Geometry: final body of the model. Coordinates: model frame, mm. A direction names the side the tool comes from. Coordinates: 2 decimals unless noted, no trailing zeros. Write each loop counter-clockwise with the first axis right and the second up, starting at its lowest first coordinate (ties: lowest second). Pieces come first, ordered by that corner, then holes.
Autodesk Inventor part; units mm, degrees
ref_plane "YZ Plane" through (0, 0, 0) normal (1, 0, 0) x (0, 1, 0)
ref_plane "XZ Plane" through (0, 0, 0) normal (0, 1, 0) x (-1, 0, 0)
ref_plane "XY Plane" through (0, 0, 0) normal (0, 0, 1) x (1, 0, 0)
sketch "Sketch1" plane through (0, 0, 0) normal (0, 0, 1) x (1, 0, 0)
  circle A0 centre (0, 0) radius 5
  line L0 (0, 0) -> (25, 0) construction
  line L1 (0, -10) -> (25, -10)
  line L2 (25, 10) -> (0, 10)
  arc A1 (0, 10) -> (0, -10) centre (0, 0) ccw
  arc A2 (25, -10) -> (25, 10) centre (25, 0) ccw construction
  line L3 (25, 10) -> (25, -10)
  point P0 (12.5, 0)
  dimension "d0" = 10
  dimension "d1" = 5
  dimension "d2" = 25
extrude "Extrusion1" add sketch "Sketch1" along normal blind 4
sketch "Sketch2" plane through (0, -10, 0) normal (0, -1, 0) x (1, 0, 0)
  line L0 (0, 4) -> (25, 4)
  line L1 (25, 4) -> (10, 4)
  line L2 (10, 4) -> (10, 19)
  line L3 (10, 19) -> (25, 19)
  line L4 (25, 19) -> (25, 4)
  line L5 (17.5, 19) -> (17.5, 4) construction
  circle A0 centre (17.5, 11.5) radius 4
  point P0 (0, 0)
  dimension "d5" = 8
  dimension "d6" = 15
  dimension "d7" = 15
extrude "Extrusion2" add sketch "Sketch2" against normal up to surface (20 mm away)
fillet "Fillet1" radius 7 2 edges at (25, 0, 19) (10, 0, 19)
properties part number "cylinder bracket"
Item 1: Set-up query: faces 4 (the flat face through (10, 0, 8)), 5 (the cylindrical face through (14.55, -0.14, 14.2)). Return all of +Z, -Z, +X, -X, +Y, -Y with unobstructed straight access to the full face (end or side cutting, diameter ignored); none if empty.
Derived:
face 4: +Z, -X, +Y, -Y
face 5: +Y, -Y
Item 2: Material intervals for probe 1 along Z at (x, y) = (17.5, 1); probe 2 along Y at (x, z) = (0, 3.1); probe 3 along Z at (x, y) = (6, -8), sorted ascending.
Derived:
probe 1: z = 0 to 7.5, 15.5 to 19
probe 2: y = -10 to -5, 5 to 10
probe 3: z = 0 to 4
Item 3: Section B-B, the plane z = 11.5. Output: boundary loops of the cut face in (x, y).
Derived:
outline: (10, -10) - (13.5, -10) - (13.5, 10) - (10, 10) - close; (21.5, -10) - (25, -10) - (25, 10) - (21.5, 10) - close
Item 4: Pull-direction query (Y, two-part tool) for faces 1 (the cylindrical face through (-1.08, 4.88, 1.97)), 2 (the flat face through (25, 0, 6)), 3 (the flat face through (15, -10, 7)); classes: released by +Y, released by -Y, zero draft, split by the parting line, or undercut.
Derived:
face 1: undercut
face 2: zero draft
face 3: released by -Y
Item 5: Section D-D, the plane y = -4.25. Output: boundary loops of the cut face in (x, z).
Derived:
outline: (-9.05, 0) - (-2.63, 0) - (-2.63, 4) - (-9.05, 4) - close; (2.63, 0) - (25, 0) - (25, 12) arc R7 ccw to (18, 19) - (17, 19) arc R7 ccw to (10, 12) - (10, 4) - (2.63, 4) - close; hole circle Ø8 at (17.5, 11.5)
Item 6: Pin query (flat end, axial travel): pin 1 (1.5 mm diameter, centred on y = 4, z = 12.5, fed in from +X); pin 2 (9 mm diameter, centred on y = -3.5, z = 8, fed in from -X); pin 3 (10 mm diameter, centred on y = 7, z = 2, fed in from -X); pin 4 (6 mm diameter, centred on x = -3.5, y = 1.5, fed in from +Z). Return the tip coordinate at first contact, or that it passes through.
Derived:
pin 1: stops at x = 25
pin 2: stops at x = -9.9
pin 3: stops at x = -9.8
pin 4: stops at z = 4
Item 7: Section A-A, the plane y = 0. Output: boundary loops of the cut face in (x, z).
Derived:
outline: (-10, 0) - (-5, 0) - (-5, 4) - (-10, 4) - close; (5, 0) - (25, 0) - (25, 12) arc R7 ccw to (18, 19) - (17, 19) arc R7 ccw to (10, 12) - (10, 4) - (5, 4) - close; hole circle Ø8 at (17.5, 11.5)
Item 8: Section C-C, the plane x = 17.5. Output: boundary loops of the cut face in (y, z), plus the area to 3 significant figures.
Derived:
outline: (-10, 0) - (10, 0) - (10, 7.5) - (-10, 7.5) - close; (-10, 15.5) - (10, 15.5) - (10, 19) - (-10, 19) - close
area: 220 mm2
